Read the model definition and answer for the solid it produces. Units are mm, in the model's axes. A direction names the side the tool comes from. Coordinates: 2 decimals unless noted, no trailing zeros. Write each loop counter-clockwise with the first axis right and the second up, starting at its lowest first coordinate (ties: lowest second). Pieces come first, ordered by that corner, then holes. Notation, with made-up numbers: (27.5, 80) - (86.5, 80) arc R15 cw to (86.5, 99) - close; hole circle Ø5 at (53.25, 15). An arc over 180 degrees is marked (long way). Return JSON: item names as keys, results as strings.
```python
from build123d import *

# Parameters (mm, degrees)
F1_DEPTH = 25


with BuildPart() as f1:
    # F0 (on Top) → F1 (new body)
    with BuildSketch(Plane.XY):
        with BuildLine():
            ThreePointArc((18.250306, 103.623616), (16.492946, 107.866257), (12.250306, 109.623616))
            ThreePointArc((12.250306, 109.623616), (8.007665, 99.380976), (18.250306, 103.623616))
        make_face()
        with BuildLine():
            ThreePointArc((-1.749694, 103.623616), (-3.507054, 107.866257), (-7.749694, 109.623616))
            ThreePointArc((-7.749694, 109.623616), (-11.992335, 99.380976), (-1.749694, 103.623616))
        make_face()
        with BuildLine():
            ThreePointArc((-22.999694, 103.623616), (-24.757054, 107.866257), (-28.999694, 109.623616))
            ThreePointArc((-28.999694, 109.623616), (-33.242335, 99.380976), (-22.999694, 103.623616))
        make_face()
        with BuildLine():
            ThreePointArc((-42.999694, 103.623616), (-44.757054, 107.866257), (-48.999694, 109.623616))
            ThreePointArc((-48.999694, 109.623616), (-53.242335, 99.380976), (-42.999694, 103.623616))
        make_face()
        with BuildLine():
            ThreePointArc((-66.499694, 103.623616), (-68.696394, 108.926917), (-73.999694, 111.123616))
            ThreePointArc((-73.999694, 111.123616), (-79.302995, 98.320316), (-66.499694, 103.623616))
        make_face()
        with BuildLine():
            ThreePointArc((-40.249694, -1.320904), (-50.249694, 8.679096), (-60.249694, -1.320904))
            ThreePointArc((-60.249694, -1.320904), (-50.249694, -11.320904), (-40.249694, -1.320904))
        make_face()
        with BuildLine():
            ThreePointArc((-65.249694, -26.320904), (-75.249694, -16.320904), (-85.249694, -26.320904))
            ThreePointArc((-85.249694, -26.320904), (-75.249694, -36.320904), (-65.249694, -26.320904))
        make_face()
        with BuildLine():
            ThreePointArc((-90.249694, -51.320904), (-100.249694, -41.320904), (-110.249694, -51.320904))
            ThreePointArc((-110.249694, -51.320904), (-100.249694, -61.320904), (-90.249694, -51.320904))
        make_face()
        Polygon((-120.249694, -51.320904), (-120.249694, -66.320904), (-100.249694, -66.320904), (-75.249694, -66.320904), (-50.249694, -66.320904), (-17.749694, -66.320904), (7.250306, -13.876384), (7.250306, 48.623616), (29.750306, 48.623616), (29.750306, 103.623616), (29.750306, 121.123616), (12.250306, 121.123616), (-7.749694, 121.123616), (-28.999694, 121.123616), (-48.999694, 121.123616), (-73.999694, 121.123616), (-87.749694, 121.123616), (-87.749694, 63.623616), (-50.249694, 63.623616), (-50.249694, 46.123616), (-120.249694, 46.123616), (-120.249694, -1.320904), (-120.249694, -26.320904), align=None)
        with BuildLine():
            ThreePointArc((-90.249694, -51.320904), (-100.249694, -61.320904), (-110.249694, -51.320904))
            ThreePointArc((-110.249694, -51.320904), (-100.249694, -41.320904), (-90.249694, -51.320904))
        make_face(mode=Mode.SUBTRACT)
        with BuildLine():
            ThreePointArc((-65.249694, -26.320904), (-75.249694, -36.320904), (-85.249694, -26.320904))
            ThreePointArc((-85.249694, -26.320904), (-75.249694, -16.320904), (-65.249694, -26.320904))
        make_face(mode=Mode.SUBTRACT)
        with BuildLine():
            ThreePointArc((-40.249694, -1.320904), (-50.249694, -11.320904), (-60.249694, -1.320904))
            ThreePointArc((-60.249694, -1.320904), (-50.249694, 8.679096), (-40.249694, -1.320904))
        make_face(mode=Mode.SUBTRACT)
        with BuildLine():
            ThreePointArc((-66.499694, 103.623616), (-79.302995, 98.320316), (-73.999694, 111.123616))
            ThreePointArc((-73.999694, 111.123616), (-68.696394, 108.926917), (-66.499694, 103.623616))
        make_face(mode=Mode.SUBTRACT)
        with BuildLine():
            ThreePointArc((-42.999694, 103.623616), (-53.242335, 99.380976), (-48.999694, 109.623616))
            ThreePointArc((-48.999694, 109.623616), (-44.757054, 107.866257), (-42.999694, 103.623616))
        make_face(mode=Mode.SUBTRACT)
        with BuildLine():
            ThreePointArc((-22.999694, 103.623616), (-33.242335, 99.380976), (-28.999694, 109.623616))
            ThreePointArc((-28.999694, 109.623616), (-24.757054, 107.866257), (-22.999694, 103.623616))
        make_face(mode=Mode.SUBTRACT)
        with BuildLine():
            ThreePointArc((-1.749694, 103.623616), (-11.992335, 99.380976), (-7.749694, 109.623616))
            ThreePointArc((-7.749694, 109.623616), (-3.507054, 107.866257), (-1.749694, 103.623616))
        make_face(mode=Mode.SUBTRACT)
        with BuildLine():
            ThreePointArc((18.250306, 103.623616), (8.007665, 99.380976), (12.250306, 109.623616))
            ThreePointArc((12.250306, 109.623616), (16.492946, 107.866257), (18.250306, 103.623616))
        make_face(mode=Mode.SUBTRACT)
    extrude(amount=F1_DEPTH)


solid = f1.part
```
(1) Determine the mould class of faces 4 (the face through (-65.26, -25.88, 12.32)), 5 (the face through (29.75, 84, 12)), 6 (the face through (-69, 63.624, 12)) for opening direction X: +X half, -X half, draft (parallel to the pull), parting line (faces both ways), or undercut.
Answer:
{"face 4": "undercut", "face 5": "+X half", "face 6": "draft"}
(2) Which of the six approach directions +Z, -Z, +X, -X, +Y, -Y give full straight-line access (tool end or side, diameter ignored) to faces 1 (the face through (-87.75, 93, 12)), 2 (the face through (-85, 46.124, 12)), 3 (the face through (18, 48.624, 12))?
Answer:
{"face 1": "+Z, -Z, -X, +Y", "face 2": "+Z, -Z, -X", "face 3": "+Z, -Z, +X, -Y"}
(3) Straight lines are drawn through the part: line 1 (Y direction, x = -49.5, z = 18.5); line 2 (Y direction, x = -45, z = 6); line 3 (X direction, y = -0.5, z = 17.75). For each, find the intervals that lie inside material, in ascending order. Write a range as from..to.
Answer:
{"line 1": "-66.32..-11.29, 8.65..97.64, 109.6..121.12", "line 2": "-66.32..-9.83, 7.19..99.15, 108.1..121.12", "line 3": "-120.25..-60.22, -40.28..7.25"}
(4) A cutting plane is placed at A-A (y = -31.5). Determine the outline of the cut face in (x, z).
Answer:
{"outline": "(-120.25, 0) - (-83.8, 0) - (-83.8, 25) - (-120.25, 25) - close; (-66.7, 0) - (-1.15, 0) - (-1.15, 25) - (-66.7, 25) - close"}
(5) A cutting plane is placed at B-B (x = -94.5). Determine the outline of the cut face in (y, z), and give its area (3 significant figures).
Answer:
{"outline": "(-66.32, 0) - (-59.5, 0) - (-59.5, 25) - (-66.32, 25) - close; (-43.14, 0) - (46.12, 0) - (46.12, 25) - (-43.14, 25) - close", "area": "2,400 mm²"}
(6) Flat-ended cylindrical pins translate along their axes: P1, Ø9.5, axis at x = -7.75, y = 103.62, coming from the +Z side; P2, Ø19, axis at x = -29, y = 103.62, coming from the -Z side; P3, Ø11, axis at x = 17, z = 17.5, coming from the -Y side; P4, Ø10, axis at y = -16.5, z = 15, coming from the +X side. Find the tip coordinate at first contact, or state that the pin passes through.
Answer:
{"P1": "through", "P2": "z = 0", "P3": "y = 48.62", "P4": "x = 7.25"}
(7) A cutting plane is placed at D-D (x = -71.5). Determine the outline of the cut face in (y, z).
Answer:
{"outline": "(-66.32, 0) - (-35.59, 0) - (-35.59, 25) - (-66.32, 25) - close; (-17.05, 0) - (46.12, 0) - (46.12, 25) - (-17.05, 25) - close; (63.62, 0) - (96.55, 0) - (96.55, 25) - (63.62, 25) - close; (110.69, 0) - (121.12, 0) - (121.12, 25) - (110.69, 25) - close"}
(8) A cutting plane is placed at C-C (z = 2). State how many separate pieces and enclosed holes the cut face has, and give its area (3 significant figures).
Answer:
{"separate pieces": "1", "enclosed holes": "8", "area": "20,200 mm²"}
